Could you check a few things on this drawing? It's one solid part, dimensions in mm from its lowest x, y, z. A direction names the side the tool comes from. Give positions to 0.01 mm unless a question says otherwise; leave off trailing zeros. Write each loop counter-clockwise with the first axis right and the second up, starting at its lowest first coordinate (ties: lowest second). Pieces come first, ordered by that corner, then holes. Notation, with made-up numbers: M 43.25,31.5 L 62.25,31.5 A24 ccw 62.25,58.5 Z; hole C 14.25,-17 d10. An arc over 180 degrees is marked long. Write each question's results on one line, items separated by ' | '.
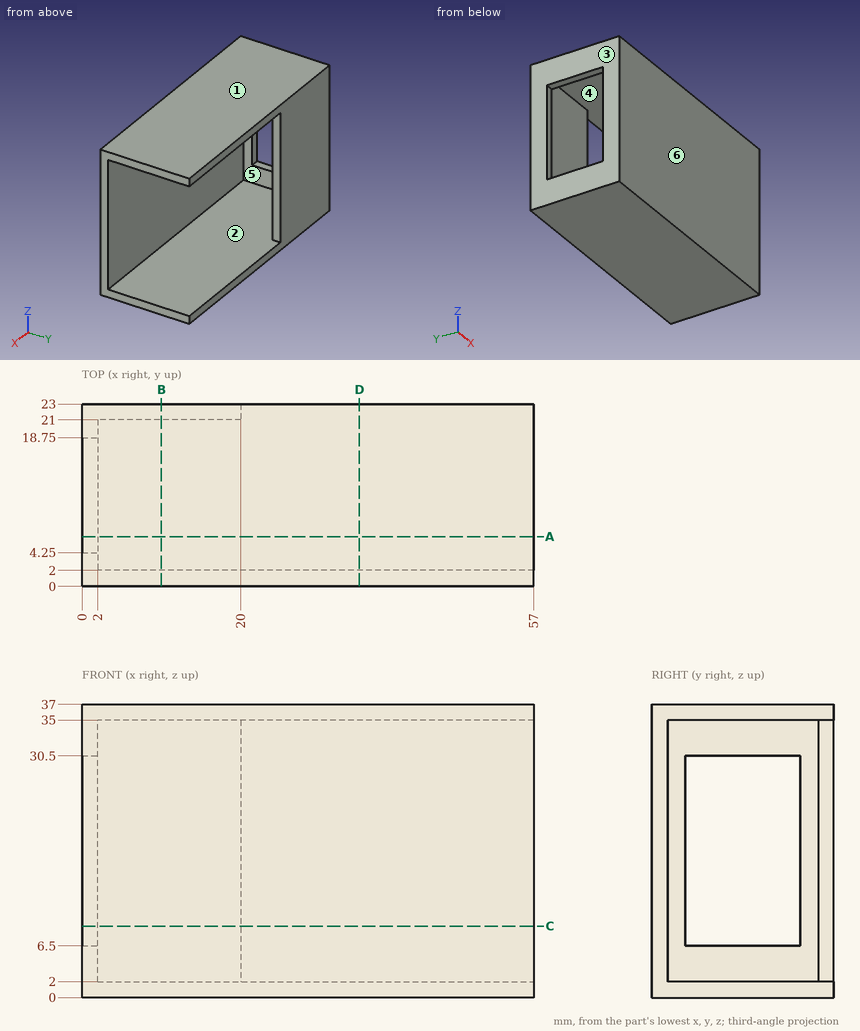
Item 1: If I drill on line 1 (Z direction, x = 8, y = 20); line 2 (Y direction, x = 6, z = 12.5); line 3 (Y direction, x = 47.5, z = 20.5), over which ranges is the centre line in solid material (lowest first)? Write a range as from..to.
Geometry says:
line 1: z = 0..2, 35..37 | line 2: y = 0..2, 21..23 | line 3: y = 0..2
Item 2: I'm going to push flat-ended pins straight in: pin 1 (1.6 mm diameter, centred on y = 22, z = 26, fed in from +X); pin 2 (4 mm diameter, centred on x = 36, z = 8.5, fed in from +Y). Where does each tip first touch, or does it pass through?
Geometry says:
pin 1: stops at x = 20 | pin 2: stops at y = 2
Item 3: I want a section at B-B, the plane x = 10. Please give me the cut outline in (y, z).
Geometry says:
outline: M 0,0 L 23,0 L 23,37 L 0,37 Z; hole M 2,2 L 21,2 L 21,35 L 2,35 Z
Item 4: I want a section at D-D, the plane x = 35. Please give me the cut outline in (y, z).
Geometry says:
outline: M 0,0 L 23,0 L 23,2 L 2,2 L 2,35 L 23,35 L 23,37 L 0,37 Z
Item 5: I want a section at C-C, the plane z = 9. Please give me the cut outline in (x, y).
Geometry says:
outline: M 0,0 L 57,0 L 57,2 L 2,2 L 2,4.25 L 0,4.25 Z; M 0,18.75 L 2,18.75 L 2,21 L 20,21 L 20,23 L 0,23 Z
Item 6: For the marked faces 1 and 2, which set-ups out of +Z, -Z, +X, -X, +Y, -Y let a thin tool reach every point of the face, with its end or its side?
Geometry says:
face 1: +Z, +X, -X, +Y, -Y | face 2: +X
Item 7: Thinking about a two-plate mould opening in Y: for the marked faces 3, 4, 5 and 6, which applies, +Y half, -Y half, draft (parallel to the pull), parting line (faces both ways), or undercut?
Geometry says:
face 3: draft | face 4: undercut | face 5: undercut | face 6: -Y half
Item 8: I want a section at A-A, the plane y = 6.25. Please give me the cut outline in (x, z).
Geometry says:
outline: M 0,0 L 57,0 L 57,2 L 2,2 L 2,6.5 L 0,6.5 Z; M 0,30.5 L 2,30.5 L 2,35 L 57,35 L 57,37 L 0,37 Z
